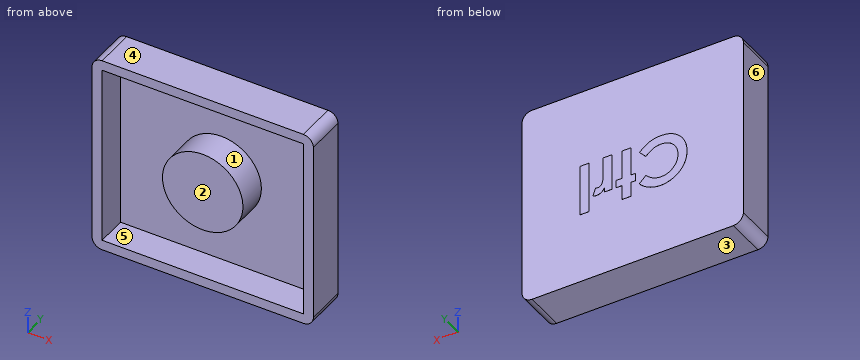
```python
from build123d import *

# Parameters (mm, degrees)
SKETCH1_W           = 13.97
SKETCH1_H           = 12.7
BOSS_EXTRUDE1_DEPTH = 2.54
FILLET1_R           = 0.635
SHELL1_START        = 0.635
SHELL1_OUTLINE_W    = 1.905
SHELL1_OUTLINE_H    = 11.43
SHELL1_DEPTH        = 12.7
SKETCH2_R           = 2.54
BOSS_EXTRUDE2_DEPTH = 1.905
SKETCH3_W           = 0.569871795
SKETCH3_H           = 3.256410256
BOSS_EXTRUDE3_DEPTH = 0.00254


# Read off the part's stored shape, not the designer's step: Shell1
with BuildPart() as part:
    # Sketch1 → Boss-Extrude1 (new body)
    with BuildSketch(Plane(origin=(0, 0, 0), x_dir=(1, 0, 0), z_dir=(0, 1, 0))):
        with Locations((6.985, 6.35)):
            Rectangle(SKETCH1_W, SKETCH1_H)
    extrude(amount=BOSS_EXTRUDE1_DEPTH)

    # Fillet1
    fillet1_edges = [part.edges().sort_by_distance(p)[0] for p in [
        (0, 1.27, -12.7),
        (13.97, 1.27, -12.7),
        (13.97, 1.27, 0),
        (0, 1.27, 0),
    ]]
    fillet(fillet1_edges, radius=FILLET1_R)

    # Shell1 outline → Shell1 (cut)
    with BuildSketch(Plane.YZ.offset(SHELL1_START)):
        with Locations((0.9525, -6.35)):
            Rectangle(SHELL1_OUTLINE_W, SHELL1_OUTLINE_H)
    extrude(amount=SHELL1_DEPTH, mode=Mode.SUBTRACT)

    # Sketch2 → Boss-Extrude2 (add)
    with BuildSketch(Plane(origin=(0, 1.905, 0), x_dir=(-1, 0, 0), z_dir=(0, -1, 0))):
        with Locations(Location((-6.985, 6.35, 0), (0, 0, 270))):
            Circle(SKETCH2_R)
    extrude(amount=BOSS_EXTRUDE2_DEPTH)

    # Sketch3 → Boss-Extrude3 (add)
    with BuildSketch(Plane(origin=(0, 2.54, 0), x_dir=(1, 0, 0), z_dir=(0, 1, 0))):
        with BuildLine():
            Line((6.568505128, 7.577208734), (6.150641546, 7.177789663))
            add(Edge.make_bspline(
                [(6.150641546, 7.177789663), (6.115194953, 7.2144415), (6.045956652, 7.28603402), (5.934387691, 7.380816208), (5.818360035, 7.459804336), (5.700130769, 7.526327635), (5.577573291, 7.576657252), (5.452104701, 7.613333291), (5.322923843, 7.635693286), (5.235499207, 7.638251666), (5.191526963, 7.639538462)],
                knots=[0, 0, 0, 0, 1.115251505, 2.178435587, 3.19620269, 4.182487026, 5.141301733, 6.088180966, 7.038406374, 8, 8, 8, 8], degree=3))
            add(Edge.make_bspline(
                [(5.191526963, 7.639538462), (5.154804796, 7.638521848), (5.082337645, 7.636515672), (4.975936877, 7.621808428), (4.874159044, 7.596798119), (4.776655743, 7.562329281), (4.683713883, 7.517728433), (4.5951386, 7.463030097), (4.511148271, 7.398728275), (4.432852361, 7.325155668), (4.361230014, 7.244772066), (4.29794711, 7.159002955), (4.244937527, 7.068044826), (4.201433425, 6.972818837), (4.16754541, 6.872884235), (4.143345111, 6.7683083), (4.129348304, 6.658966489), (4.127259187, 6.584636741), (4.126197436, 6.546860176)],
                knots=[0, 0, 0, 0, 1.035432265, 2.043311493, 3.022114605, 3.98653278, 4.95457646, 5.923598177, 6.917315552, 7.932509744, 8.948865224, 9.949768934, 10.933144597, 11.912367597, 12.897413939, 13.903909035, 14.934704909, 16, 16, 16, 16], degree=3))
            add(Edge.make_bspline(
                [(4.126197436, 6.546860176), (4.12650342, 6.52034594), (4.127106522, 6.468085836), (4.133708537, 6.390778637), (4.144339337, 6.315772378), (4.159724739, 6.243180674), (4.178964335, 6.172940615), (4.201536762, 6.104446244), (4.229853539, 6.038643999), (4.26128559, 5.974769629), (4.297840702, 5.914566028), (4.337253857, 5.857156898), (4.379990988, 5.802823652), (4.426328908, 5.751788408), (4.476919763, 5.704848731), (4.530455968, 5.660593089), (4.587840605, 5.620129351), (4.647881648, 5.582442035), (4.711097778, 5.549702743), (4.775773793, 5.52004727), (4.842890313, 5.495962616), (4.911630153, 5.476548188), (4.981747662, 5.460039117), (5.053928654, 5.449873974), (5.12754741, 5.442176031), (5.177301332, 5.441700728), (5.202339263, 5.441461538)],
                knots=[0, 0, 0, 0, 1.103660481, 2.175337485, 3.227646561, 4.255952547, 5.262355991, 6.258840057, 7.255597736, 8.242457506, 9.22035537, 10.185017736, 11.140346927, 12.096287581, 13.051739095, 14.01125915, 14.986044842, 15.97314143, 16.960198552, 17.947847494, 18.933482797, 19.925264591, 20.920966487, 21.929612487, 22.958107872, 24, 24, 24, 24], degree=3))
            add(Edge.make_bspline(
                [(5.202339263, 5.441461538), (5.244807897, 5.442689957), (5.328247719, 5.445103479), (5.450707656, 5.463976883), (5.567399775, 5.495022564), (5.66063622, 5.53168571), (5.733684512, 5.567891042), (5.789295097, 5.601379191), (5.846800776, 5.638839363), (5.905246429, 5.681685345), (5.965289454, 5.729402968), (6.025869952, 5.783037337), (6.088538796, 5.840822348), (6.129592535, 5.882064647), (6.150641546, 5.903210337)],
                knots=[0, 0, 0, 0, 1.404581149, 2.759636711, 4.088442092, 5.392261763, 6.066678138, 6.783632037, 7.538459478, 8.336747902, 9.180226004, 10.074962426, 11.012997595, 12, 12, 12, 12], degree=3))
            Line((6.150641546, 5.903210337), (6.555784776, 5.477714543))
            add(Edge.make_bspline(
                [(6.555784776, 5.477714543), (6.527305387, 5.450218588), (6.471719712, 5.396552363), (6.387870264, 5.320351332), (6.304126343, 5.251876235), (6.222511029, 5.188641725), (6.141687378, 5.132489979), (6.06166396, 5.083364915), (5.983346676, 5.04002409), (5.905109243, 5.003198427), (5.826464826, 4.971929614), (5.745548963, 4.945009219), (5.662114287, 4.922235533), (5.575651216, 4.903860159), (5.486966225, 4.88912559), (5.395229341, 4.879179841), (5.301022221, 4.872493645), (5.237120072, 4.871892834), (5.204883333, 4.871589744)],
                knots=[0, 0, 0, 0, 1.244526981, 2.429050516, 3.560637417, 4.644440555, 5.67424972, 6.652764056, 7.595344123, 8.486817594, 9.369275933, 10.254498637, 11.166417451, 12.086725134, 13.032340136, 13.991389299, 14.986715468, 16, 16, 16, 16], degree=3))
            add(Edge.make_bspline(
                [(5.204883333, 4.871589744), (5.145668437, 4.873099249), (5.029801344, 4.876052933), (4.86000114, 4.897937726), (4.698695505, 4.934627196), (4.545492012, 4.986516227), (4.400439375, 5.052802032), (4.263574704, 5.134065316), (4.135118595, 5.230090176), (4.016108719, 5.339751107), (3.908458622, 5.460862399), (3.813308403, 5.590902701), (3.734600139, 5.730511114), (3.669246971, 5.877625175), (3.618141653, 6.032916222), (3.582172173, 6.196552234), (3.559990057, 6.36837521), (3.557563302, 6.485734263), (3.556325641, 6.545588141)],
                knots=[0, 0, 0, 0, 1.078019885, 2.10938526, 3.111377082, 4.085535484, 5.04941344, 6.010039228, 6.978205633, 7.964457913, 8.951525778, 9.924444315, 10.892603023, 11.863865945, 12.85144698, 13.863884204, 14.910567087, 16, 16, 16, 16], degree=3))
            add(Edge.make_bspline(
                [(3.556325641, 6.545588141), (3.556848616, 6.58462433), (3.557885026, 6.661984515), (3.568777786, 6.775942336), (3.583962928, 6.887030827), (3.608052774, 6.994096523), (3.637090707, 7.098581794), (3.673203193, 7.199351009), (3.716332553, 7.296693788), (3.765088628, 7.390773089), (3.820245888, 7.480972592), (3.881862603, 7.56651734), (3.948352517, 7.648067724), (4.021313276, 7.724541827), (4.099684664, 7.796611105), (4.183820519, 7.863885002), (4.273214805, 7.927328301), (4.36810948, 7.985304953), (4.466660994, 8.037747916), (4.567626351, 8.08400485), (4.670757492, 8.122664994), (4.775618369, 8.154732158), (4.882652019, 8.178668028), (4.991094461, 8.19678671), (5.101868412, 8.206915169), (5.176243523, 8.208573262), (5.21378758, 8.209410256)],
                knots=[0, 0, 0, 0, 1.071919942, 2.124283339, 3.142214191, 4.149696895, 5.136002878, 6.119640489, 7.086990633, 8.058538607, 9.028339693, 9.988281803, 10.952401235, 11.916291999, 12.888973767, 13.874849856, 14.873389453, 15.898127285, 16.927174885, 17.938320013, 18.946391617, 19.950418109, 20.947802303, 21.956882652, 22.968648068, 24, 24, 24, 24], degree=3))
            add(Edge.make_bspline(
                [(5.21378758, 8.209410256), (5.24581651, 8.20893047), (5.309541359, 8.207975887), (5.404438353, 8.200018393), (5.498576405, 8.187521229), (5.591618472, 8.168665671), (5.684230086, 8.14628174), (5.775194226, 8.11697307), (5.865945903, 8.084303034), (5.955061809, 8.045252678), (6.042666337, 8.002625686), (6.126707215, 7.954263816), (6.20859548, 7.903143202), (6.286516537, 7.846238304), (6.361930016, 7.785613168), (6.434441572, 7.720984943), (6.503414876, 7.651276087), (6.546698691, 7.602022665), (6.568505128, 7.577208734)],
                knots=[0, 0, 0, 0, 0.996412454, 1.982464992, 2.961075852, 3.949442424, 4.934965278, 5.923860011, 6.921385422, 7.934793307, 8.949617135, 9.951082467, 10.950285876, 11.951772932, 12.951063433, 13.960125323, 14.972308753, 16, 16, 16, 16], degree=3))
        make_face()
        Polygon((7.097671795, 8.209410256), (7.66754359, 8.209410256), (7.66754359, 7.273192308), (8.033889744, 7.273192308), (8.033889744, 6.784730769), (7.66754359, 6.784730769), (7.66754359, 4.953), (7.097671795, 4.953), (7.097671795, 6.784730769), (6.812735897, 6.784730769), (6.812735897, 7.273192308), (7.097671795, 7.273192308), align=None)
        with BuildLine():
            Line((8.278120513, 7.273192308), (8.766582051, 7.273192308))
            Line((8.766582051, 7.273192308), (8.766582051, 6.987620393))
            add(Edge.make_bspline(
                [(8.766582051, 6.987620393), (8.78039969, 7.012999247), (8.80740684, 7.062603272), (8.857021237, 7.129186851), (8.914020267, 7.185261684), (8.976355778, 7.232000626), (9.044216695, 7.268429043), (9.115785825, 7.294388882), (9.190450896, 7.31125918), (9.241384876, 7.313011685), (9.267127925, 7.313897436)],
                knots=[0, 0, 0, 0, 1.09866127, 2.147379032, 3.14564304, 4.131443017, 5.102343063, 6.064490016, 7.021754664, 8, 8, 8, 8], degree=3))
            add(Edge.make_bspline(
                [(9.267127925, 7.313897436), (9.28582059, 7.313022129), (9.323885533, 7.311239691), (9.381901861, 7.300878355), (9.440755263, 7.282143087), (9.479485873, 7.265274469), (9.499274359, 7.256655849)],
                knots=[0, 0, 0, 0, 0.931404136, 1.896671404, 2.925354185, 4, 4, 4, 4], degree=3))
            Line((9.499274359, 7.256655849), (9.322461458, 6.77391847))
            add(Edge.make_bspline(
                [(9.322461458, 6.77391847), (9.30665691, 6.781554463), (9.276950443, 6.795907192), (9.233821811, 6.81284489), (9.194680789, 6.823179446), (9.1698661, 6.824721452), (9.15836891, 6.825435897)],
                knots=[0, 0, 0, 0, 1.214386998, 2.282580073, 3.20428172, 4, 4, 4, 4], degree=3))
            add(Edge.make_bspline(
                [(9.15836891, 6.825435897), (9.147513328, 6.824962468), (9.126158527, 6.824031151), (9.094639437, 6.816050083), (9.064955019, 6.802286977), (9.035674781, 6.784655073), (9.009108609, 6.760145407), (8.982558846, 6.731771118), (8.959161774, 6.696739283), (8.934471077, 6.657747072), (8.913447831, 6.610020641), (8.895421046, 6.553045117), (8.879359035, 6.486161255), (8.868306178, 6.409013934), (8.857623149, 6.322349687), (8.851264348, 6.225532411), (8.846525052, 6.118868249), (8.846235276, 6.044412815), (8.846084255, 6.005609175)],
                knots=[0, 0, 0, 0, 0.544232178, 1.070598461, 1.618251235, 2.182094276, 2.777567932, 3.425210017, 4.127676488, 4.886675562, 5.738955394, 6.734782583, 7.883056018, 9.186093582, 10.642914445, 12.264202625, 14.053029461, 16, 16, 16, 16], degree=3))
            Line((8.846084255, 6.005609175), (8.847992308, 5.892398037))
            Line((8.847992308, 5.892398037), (8.847992308, 4.953))
            Line((8.847992308, 4.953), (8.278120513, 4.953))
            Line((8.278120513, 4.953), (8.278120513, 7.273192308))
        make_face()
        with Locations((10.028441026, 6.581205128)):
            Rectangle(SKETCH3_W, SKETCH3_H)
    extrude(amount=BOSS_EXTRUDE3_DEPTH)


solid = part.part
```
CAD build for the part. Positions are in the model's coordinates, mm. Face numbers are marked on the shaded views. A direction names the side the tool comes from. Coordinates: 2 decimals unless noted, no trailing zeros. Order: outer loops, then holes, each group sorted by start corner. A loop starts at its lowest first (then second) coordinate and runs counter-clockwise, first axis right, second up. Notation, with made-up numbers: M 40.25,2.25 L 94.25,2.25 A20 ccw 94.25,13.25 Z; hole C -2.5,-20 d6. An arc over 180 degrees is marked long. Answer as CSV lines item,"result".
1) Drill centre lines: L1, parallel to X at y = 1.85, z = -12 (3 decimals); L2, parallel to Z at x = 4, y = 1.7 (3 decimals); L3, parallel to Z at x = 5, y = 1.85 (3 decimals). Where is each one in solid material? Low to high. Write a range as from..to.
Verdict:
L1,"0..0.635, 13.335..13.97"
L2,"-12.7..-12.065, -0.635..0"
L3,"-12.7..-12.065, -7.935..-4.765, -0.635..0"
2) Flat gauge pin, fed straight in: P1, Ø6, axis at x = 4.5, z = -3.5, coming from the -Y side. Where does the tip first touch, or does it go through?
Verdict:
P1,"y = 0"
3) Cut at B-B (z = -1.5). List the corners of the cut face in (x, y) (3 decimals), then the cut area to 3 significant figures.
Verdict:
outline,"M 0,0 L 0.635,0 L 0.635,1.905 L 13.335,1.905 L 13.335,0 L 13.97,0 L 13.97,2.54 L 0,2.54 Z"
area,"11.3 mm2"
4) 3-axis set-ups, long thin cutter, end or side, ignore diameter. For the marked faces 5 and 6: which of +Z, -Z, +X, -X, +Y, -Y reach the whole face in a straight line?
Verdict:
face 5,"-Y"
face 6,"+Z, -Z, -X, +Y, -Y"
5) Cut at A-A (y = 0.2). List the corners of the cut face in (x, z) (3 decimals), then the cut area to 3 significant figures.
Verdict:
outline,"M 0,-12.065 A0.635 ccw 0.635,-12.7 L 13.335,-12.7 A0.635 ccw 13.97,-12.065 L 13.97,-0.635 A0.635 ccw 13.335,0 L 0.635,0 A0.635 ccw 0,-0.635 Z; C 6.985,-6.35 d5.08; hole M 0.635,-12.065 L 13.335,-12.065 L 13.335,-0.635 L 0.635,-0.635 Z"
area,"52.2 mm2"
6) Mould opens along Z. For the marked faces 1, 2, 3 and 4 say: released by +Z, released by -Z, zero draft, split by the parting line, or undercut.
Verdict:
face 1,"undercut"
face 2,"zero draft"
face 3,"released by -Z"
face 4,"released by +Z"
